from build123d import *

# Parameters (mm, degrees)
SKETCH1_R           = 19.05
EXTRUDE1_DEPTH      = 19.05
EXTRUDE1_DEPTH_BACK = 50.8
CUT_EXTRUDE1_REACH  = 52.8
SKETCH2_R           = 19.05
SKETCH2_R_2         = 13.3604
CUT_EXTRUDE3_REACH  = 21.05
SKETCH19_R          = 8.6614
CUT_EXTRUDE4_DEPTH  = 0.254
SKETCH20_R          = 8.6614
CUT_EXTRUDE5_DEPTH  = 0.254
CHAMFER1_SIZE       = 0.762
SKETCH15_R          = 5.3086
EXTRUDE2_DEPTH      = 1.27
CIRPATTERN1_COUNT   = 4


with BuildPart() as part:
    # Sketch1 → Extrude1 (new body, two sides)
    with BuildSketch(Plane(origin=(0, 0, 0), x_dir=(0, 0, -1), z_dir=(1, 0, 0))) as extrude1_sk:
        Circle(SKETCH1_R)
    extrude(amount=EXTRUDE1_DEPTH)
    extrude(extrude1_sk.sketch, amount=-EXTRUDE1_DEPTH_BACK)

    # Sketch2 → Cut-Extrude1 (cut, up to next)
    with BuildSketch(Plane(origin=(0, 0, 0), x_dir=(0, 0, -1), z_dir=(1, 0, 0)), mode=Mode.PRIVATE) as cut_extrude1_sk1:
        Circle(SKETCH2_R)
        with Locations((0, -4.7498)):
            Circle(SKETCH2_R_2, mode=Mode.SUBTRACT)
    cut_extrude1_tool1 = extrude(cut_extrude1_sk1.sketch, amount=-CUT_EXTRUDE1_REACH, mode=Mode.PRIVATE) & part.part
    add(cut_extrude1_tool1.solids().sort_by_distance((0, 0, 18.511185))[0], mode=Mode.SUBTRACT)

    # Sketch4 → Cut-Extrude3 (cut, up to next)
    with BuildSketch(Plane.ZY, mode=Mode.PRIVATE) as cut_extrude3_sk1:
        with BuildLine():
            Line((14.2875, -12.600390619), (14.2875, 11.344778237))
            Line((14.2875, 11.344778237), (0, 18.007148903))
            Line((0, 18.007148903), (-14.2875, 11.344778237))
            Line((-14.2875, 11.344778237), (-14.2875, -12.600390619))
            ThreePointArc((-14.2875, -12.600390619), (0, 19.05), (14.2875, -12.600390619))
        make_face()
    cut_extrude3_tool1 = extrude(cut_extrude3_sk1.sketch, amount=-CUT_EXTRUDE3_REACH, mode=Mode.PRIVATE) & part.part
    add(cut_extrude3_tool1.solids().sort_by_distance((0, -0.627806, 14.782814))[0], mode=Mode.SUBTRACT)

    # Sketch6 → Cut-Revolve2 (revolve, cut)
    with BuildSketch(Plane.XY, mode=Mode.PRIVATE) as cut_revolve2_sk:
        Polygon((12.169188023, 18.007148903), (19.05, 3.2512), (19.05, 18.007148903), align=None)
    revolve(cut_revolve2_sk.sketch.rotate(Axis((1.987224567, -4.7498, 0), (1, 0, 0)), 270), axis=Axis((1.987224567, -4.7498, 0), (1, 0, 0)), mode=Mode.SUBTRACT)  # turned: the seam where the file's is

    # S2D0002 → Cut-Revolve3 (revolve, cut)
    with BuildSketch(Plane(origin=(6.35, 13.712414668, 8.609072086), x_dir=(0, 0.422618262, -0.906307787), z_dir=(1, 0, 0))):
        Polygon((0, 0), (4.5466, 0), (4.106586662, -2.0701), (3.4544, -2.722286662), (3.4544, -12.192), (0, -12.192), align=None)
    revolve(axis=Axis((6.35, 2.110224902, 3.198882147), (0, 0.906307787, 0.422618262)), mode=Mode.SUBTRACT)

    # Sketch19 → Cut-Extrude4 (cut)
    with BuildSketch(Plane(origin=(0, 14.790960552, 6.897138177), x_dir=(1, 0, 0), z_dir=(0, 0.906307787, 0.422618262))):
        with Locations((6.35, -2.00735222)):
            Circle(SKETCH19_R)
    extrude(amount=-CUT_EXTRUDE4_DEPTH, mode=Mode.SUBTRACT)

    # Sketch8 → Cut-Revolve4 (revolve, cut)
    with BuildSketch(Plane(origin=(6.35, 13.712414668, -8.609072086), x_dir=(0, -0.422618262, -0.906307787), z_dir=(1, 0, 0))):
        Polygon((0, 0), (4.5466, 0), (4.106586662, -2.0701), (3.4544, -2.722286662), (3.4544, -12.192), (0, -12.192), align=None)
    revolve(axis=Axis((6.35, 2.110224902, -3.198882147), (0, 0.906307787, -0.422618262)), mode=Mode.SUBTRACT)

    # Sketch20 → Cut-Extrude5 (cut)
    with BuildSketch(Plane(origin=(0, 14.790960552, -6.897138177), x_dir=(1, 0, 0), z_dir=(0, 0.906307787, -0.422618262))):
        with Locations((6.35, 2.00735222)):
            Circle(SKETCH20_R)
    extrude(amount=-CUT_EXTRUDE5_DEPTH, mode=Mode.SUBTRACT)

    # Sketch10 → Cut-Revolve6 (revolve, cut)
    with BuildSketch(Plane.XY, mode=Mode.PRIVATE) as cut_revolve6_sk:
        Polygon((0, 8.6106), (0, 7.5692), (-3.81, 7.5692), (-4.8514, 8.6106), align=None)
    revolve(cut_revolve6_sk.sketch.rotate(Axis((-5.09397, -4.7498, 0), (1, 0, 0)), 90), axis=Axis((-5.09397, -4.7498, 0), (1, 0, 0)), mode=Mode.SUBTRACT)  # turned: the seam where the file's is

    # Sketch12 → Cut-Revolve8 (revolve, cut)
    with BuildSketch(Plane.XY, mode=Mode.PRIVATE) as cut_revolve8_sk:
        Polygon((-50.8, 8.6106), (-50.8, 7.5692), (-49.276, 7.5692), (-48.2346, 8.6106), align=None)
    revolve(cut_revolve8_sk.sketch.rotate(Axis((-50.92827, -4.7498, 0), (1, 0, 0)), 90), axis=Axis((-50.92827, -4.7498, 0), (1, 0, 0)), mode=Mode.SUBTRACT)  # turned: the seam where the file's is

    # Chamfer1
    chamfer1_edges = [part.edges().sort_by_distance(p)[0] for p in [
        (-50.8, -4.7498, -12.319),
    ]]
    chamfer(chamfer1_edges, length=CHAMFER1_SIZE)

    # Sketch13 → Revolve1 (revolve)
    with BuildSketch(Plane(origin=(0, 0, 0), x_dir=(0, -1, 0), z_dir=(0, 0, 1)), mode=Mode.PRIVATE) as revolve1_sk:
        with BuildLine():
            Line((4.7498, 19.05), (4.7498, 39.3192))
            Line((4.7498, 39.3192), (9.29005, 39.3192))
            ThreePointArc((9.29005, 39.3192), (10.00847049, 39.02162049), (10.30605, 38.3032))
            Line((10.30605, 38.3032), (10.30605, 19.05))
            Line((10.30605, 19.05), (4.7498, 19.05))
        make_face()
    revolve(revolve1_sk.sketch.rotate(Axis((18.03654, -4.7498, 0), (1, 0, 0)), 270), axis=Axis((18.03654, -4.7498, 0), (1, 0, 0)))  # turned: the seam where the file's is

    # S2D0001 → Cut-Revolve9 (revolve, cut)
    with BuildSketch(Plane(origin=(39.3192, -7.5565, 0), x_dir=(0, -1, 0), z_dir=(0, 0, 1)), mode=Mode.PRIVATE) as cut_revolve9_sk:
        Polygon((0, 0), (0, -10.16), (-2.8067, -11.846435499), (-2.8067, 0), align=None)
    revolve(cut_revolve9_sk.sketch.rotate(Axis((26.880442726, -4.7498, 0), (1, 0, 0)), 270), axis=Axis((26.880442726, -4.7498, 0), (1, 0, 0)), mode=Mode.SUBTRACT)  # turned: the seam where the file's is

    # Sketch15 → Extrude2 (add)
    with BuildSketch(Plane(origin=(19.05, 14.560758374, -6.789793138), x_dir=(0, -0.422618262, -0.906307787), z_dir=(0, -0.906307787, 0.422618262))):
        with Locations((2.00735222, -12.7)):
            Circle(SKETCH15_R)
    extrude(amount=-EXTRUDE2_DEPTH)

    # Sketch16 → Cut-Revolve10 (revolve, cut)
    with BuildSketch(Plane(origin=(35.3568, -0.820937947, -3.928862053), x_dir=(-1, 0, 0), z_dir=(0, -0.707106781, -0.707106781)), mode=Mode.PRIVATE) as cut_revolve10_sk:
        Polygon((0, 0), (1.5875, 0), (0, -1.5875), align=None)
    cut_revolve10 = revolve(cut_revolve10_sk.sketch.rotate(Axis((35.3568, -3.280818463, -1.468981537), (0, 0.707106781, -0.707106781)), 90), axis=Axis((35.3568, -3.280818463, -1.468981537), (0, 0.707106781, -0.707106781)), mode=Mode.SUBTRACT)  # turned: the seam where the file's is

    # CirPattern1: Cut-Revolve10 ×4 about axis
    cirpattern1_axis = Axis((18.03654, -4.7498, 0), (-1, 0, 0))
    for i in range(1, CIRPATTERN1_COUNT):
        add(cut_revolve10.rotate(cirpattern1_axis, i * 360 / CIRPATTERN1_COUNT), mode=Mode.SUBTRACT)


solid = part.part
The listing builds one solid part. Answer for the finished solid, in the listing's coordinates (mm). A direction names the side the tool comes from. Round coordinates to 2 decimals unless told otherwise and drop trailing zeros. Order: outer loops, then holes, each group sorted by start corner. A loop starts at its lowest first (then second) coordinate and runs counter-clockwise, first axis right, second up. Notation, with made-up numbers: (37, 51) -> (67, 51) arc R27 cw to (67, 70) -> close; hole circle Ø8 at (4.25, -34.75). An arc over 180 degrees is marked (long way). Write each question's results on one line, items separated by ' | '. Start each with the question number.
Q1. Which of the six approach directions +Z, -Z, +X, -X, +Y, -Y give full straight-line access (tool end or side, diameter ignored) to faces 1 (the flat face through (8, 0, -14.288)), 2 (the cylindrical face through (-49.652, 7.276, -2.671)), 3 (the flat face through (0, 8, 0))?
Q2. Each of these flat-tipped pins is pushed along its axis until it touches: pin 1 (12 mm diameter, centred on x = 26, y = 13, fed in from -Z); pin 2 (12 mm diameter, centred on x = -34, z = -8, fed in from +Y); pin 3 (2 mm diameter, centred on y = 12.5, z = -2, fed in from +X); pin 4 (1 mm diameter, centred on x = -4, z = -8, fed in from +Y). Where does it stop, or does it pass through?
Q3. Find section A-A (x = -20). Determine the outline of the cut face in (y, z).
Q4. The mould has two halves that part along Z. Classify faces 4 (the cylindrical face through (34.17, -2.01, -0.61)), 5 (the cylindrical face through (9.722, 7.21, -4.751)), 6 (the conical face through (35.19, -1.36, -2.83)), 7 (the conical face through (18.72, 3.89, 1.13)): pulls with the +Z half, pulls with the -Z half, needs draft (parallel to the pull), parting line crosses it, or undercut.
Q5. Straight lines are drawn through the part: probe 1 along Y at (x, z) = (31.75, 0); probe 2 along X at (y, z) = (6.5, -5.75); probe 3 along X at (y, z) = (-12.5, 8). For each, find the intervals that lie inside material, in ascending order. Write a range as from..to.
Worked answers:
1) face 1: -Z, +X, -X, +Y, -Y | face 2: -X | face 3: none
2) pin 1: passes through | pin 2: stops at y = 8.46 | pin 3: stops at x = 15.15 | pin 4: stops at y = 5.62
3) outline: circle Ø26.72 at (-4.75, 0)
4) face 4: undercut | face 5: undercut | face 6: pulls with the -Z half | face 7: parting line crosses it
5) probe 1: y = -10.31..-7.56, -1.94..0.81 | probe 2: x = -48.96..-4.13, 0..2.93, 9.77..16.89 | probe 3: x = -50.8..17.59
